Geometry check sheet. Reference: the model listing, model coordinates, mm. A direction names the side the tool comes from. Round coordinates to 2 decimals unless told otherwise and drop trailing zeros. Write each loop counter-clockwise with the first axis right and the second up, starting at its lowest first coordinate (ties: lowest second). Pieces come first, ordered by that corner, then holes. Notation, with made-up numbers: (-11.75, 13) - (16.25, 13) arc R21 ccw to (16.25, 47) - close; hole circle Ø2 at (-4.75, 41.5). An arc over 180 degrees is marked (long way). Return JSON: item names as keys, results as strings. Group by question number.
from build123d import *

# Parameters (mm, degrees)
CROQUIS1_R              = 7.5
CROQUIS2_R              = 7.5
SALIENTE_EXTRUIR1_DEPTH = 300


with BuildPart() as part:
    # Barrer1: sweep along a curve in space
    with BuildLine() as barrer1_path:
        Line((0, 0, 0), (0, 0, 30))
        ThreePointArc((0, 0, 30), (0, 2.928932188, 37.071067812), (0, 10, 40))
        Line((0, 10, 40), (0, 60, 40))
        ThreePointArc((0, 60, 40), (0, 67.071067812, 42.928932188), (0, 70, 50))
        Line((0, 70, 50), (0, 70, 80))
    # Croquis1 → Barrer1 (sweep)
    with BuildSketch(Plane.XY):
        Circle(CROQUIS1_R)
    sweep(path=barrer1_path.line)

    # Croquis2 → Saliente-Extruir1 (add)
    with BuildSketch(Plane(origin=(0, 0, 0), x_dir=(-1, 0, 0), z_dir=(0, 0, -1))):
        Circle(CROQUIS2_R)
    extrude(amount=SALIENTE_EXTRUIR1_DEPTH)


solid = part.part
1. Section check B-B (z = -107.5). Enter the section's corners in (x, y), and give its area (3 significant figures).
2. Section check A-A (x = 0). Enter the section's corners in (y, z), and give its area (3 significant figures).
3. Tool access check on faces 1 (the face through (-1.63, 62.68, 65.21)), 2 (the face through (-1.63, 35.35, 47.32)), 3 (the face through (0, 0, -300)). Record the directions out of +Z, -Z, +X, -X, +Y, -Y that give a thin tool (end or side, any length) a straight path to the whole face; none if there is none.
4. Section check C-C (y = 36.5). Enter the section's corners in (x, z), and give its area (3 significant figures).
5. Depth check by flat-ended pin: pin 1 Ø6 at (x, z) = (3.5, -55.5) entering from +Y; pin 2 Ø8 at (x, y) = (-0.5, 57) entering from +Z; pin 3 Ø3 at (x, y) = (-3, 45) entering from +Z. Enter the tip coordinate at first touch or a pass-through.
6. Material ranges on line 1 along Z through (x, y) = (-0.5, 12); line 2 along Y through (x, z) = (-1, 16); line 3 along Z through (x, y) = (5, 61), recorded low to high.
Result sheet:
{
 "1": {"outline": "circle Ø15 at (0, 0)", "area": "177 mm²"},
 "2": {"outline": "(-7.5, -300) - (7.5, -300) - (7.5, 30) arc R2.5 cw to (10, 32.5) - (60, 32.5) arc R17.5 ccw to (77.5, 50) - (77.5, 80) - (62.5, 80) - (62.5, 50) arc R2.5 cw to (60, 47.5) - (10, 47.5) arc R17.5 ccw to (-7.5, 30) - close", "area": "6,620 mm²"},
 "3": {"face 1": "+Z", "face 2": "none", "face 3": "-Z, +X, -X, +Y, -Y"},
 "4": {"outline": "circle Ø15 at (0, 40)", "area": "177 mm²"},
 "5": {"pin 1": "stops at y = 7.48", "pin 2": "stops at z = 47.7", "pin 3": "stops at z = 47.35"},
 "6": {"line 1": "z = 32.52 to 47.48", "line 2": "y = -7.43 to 7.43", "line 3": "z = 34.44 to 45.71"}
}
